```python
from build123d import *

# Parameters (mm, degrees)
SKETCH1_W           = 80
SKETCH1_H           = 80
BOSS_EXTRUDE1_DEPTH = 14
FILLET1_R           = 2
FILLET2_R           = 4
SKETCH2_R           = 5.75
CUT_EXTRUDE1_DEPTH  = 2
SKETCH3_R           = 1.5
CUT_EXTRUDE2_DEPTH  = 12
SKETCH6_R           = 6
CUT_EXTRUDE3_DEPTH  = 2
SKETCH7_W           = 33.5
SKETCH7_H           = 42
BOSS_EXTRUDE2_DEPTH = 2.5


with BuildPart() as part:
    # Sketch1 → Boss-Extrude1 (new, symmetric)
    with BuildSketch(Plane.XY):
        Rectangle(SKETCH1_W, SKETCH1_H)
    extrude(amount=BOSS_EXTRUDE1_DEPTH, both=True)

    # Fillet1
    fillet1_edges = [part.edges().sort_by_distance(p)[0] for p in [
        (-40, 0, 14),
        (0, -40, 14),
        (40, 0, 14),
        (0, 40, 14),
    ]]
    fillet(fillet1_edges, radius=FILLET1_R)

    # Fillet2
    # the kernel refuses this fillet: 4 mm, written as the material it takes off along each edge
    with BuildSketch(Plane(origin=(-36, -36, 14), x_dir=(-1, 0, 0), z_dir=(0, 1, 0))) as fillet2_piece_1:
        with BuildLine():
            CenterArc((2, -2), 2, 0, 90)
            Line((4, -2), (4, 0))
            Line((4, 0), (2, 0))
        make_face()
    revolve(axis=Axis((-36, -36, 14), (0, 0, 1)), revolution_arc=90, mode=Mode.SUBTRACT)
    with BuildSketch(Plane(origin=(-36, 36, 14), x_dir=(0, 1, 0), z_dir=(1, 0, 0))) as fillet2_piece_2:
        with BuildLine():
            CenterArc((2, -2), 2, 0, 90)
            Line((4, -2), (4, 0))
            Line((4, 0), (2, 0))
        make_face()
    revolve(axis=Axis((-36, 36, 14), (0, 0, 1)), revolution_arc=90, mode=Mode.SUBTRACT)
    with BuildSketch(Plane(origin=(36, -36, 14), x_dir=(0, -1, 0), z_dir=(-1, 0, 0))) as fillet2_piece_3:
        with BuildLine():
            CenterArc((2, -2), 2, 0, 90)
            Line((4, -2), (4, 0))
            Line((4, 0), (2, 0))
        make_face()
    revolve(axis=Axis((36, -36, 14), (0, 0, 1)), revolution_arc=90, mode=Mode.SUBTRACT)
    with BuildSketch(Plane(origin=(36, 36, 14), x_dir=(1, 0, 0), z_dir=(0, -1, 0))) as fillet2_piece_4:
        with BuildLine():
            CenterArc((2, -2), 2, 0, 90)
            Line((4, -2), (4, 0))
            Line((4, 0), (2, 0))
        make_face()
    revolve(axis=Axis((36, 36, 14), (0, 0, 1)), revolution_arc=90, mode=Mode.SUBTRACT)
    with BuildSketch(Plane(origin=(40, 40, 14), x_dir=(-1, 0, 0), z_dir=(0, 0, -1)), Plane(origin=(40, -40, 14), x_dir=(0, 1, 0), z_dir=(0, 0, -1)), Plane(origin=(-40, -40, -24), x_dir=(0, 1, 0), z_dir=(0, 0, 1)), Plane(origin=(-40, 40, -24), x_dir=(1, 0, 0), z_dir=(0, 0, 1))) as fillet2_piece_5:
        with BuildLine():
            CenterArc((FILLET2_R, -FILLET2_R), FILLET2_R, 90, 90)
            Line((0, -FILLET2_R), (0, 0))
            Line((0, 0), (FILLET2_R, 0))
        make_face()
    extrude(amount=38, mode=Mode.SUBTRACT)

    # Sketch2 → Cut-Extrude1 (cut)
    with BuildSketch(Plane.XY.offset(14)):
        with Locations((-27.6, 30.4)):
            Circle(SKETCH2_R)
        with Locations((-11.8, 30.4)):
            Circle(SKETCH2_R)
        with Locations((7.5, 30.4)):
            Circle(SKETCH2_R)
        with Locations((23.3, 30.4)):
            Circle(SKETCH2_R)
    extrude(amount=-CUT_EXTRUDE1_DEPTH, mode=Mode.SUBTRACT)

    # Sketch3 → Cut-Extrude2 (cut)
    with BuildSketch(Plane.XY.offset(14)):
        with Locations((-33.45, 21.95)):
            Circle(SKETCH3_R)
        with Locations((33.55, 21.95)):
            Circle(SKETCH3_R)
        with Locations((-33.45, -33.05)):
            Circle(SKETCH3_R)
        with Locations((33.55, -33.05)):
            Circle(SKETCH3_R)
    extrude(amount=-CUT_EXTRUDE2_DEPTH, mode=Mode.SUBTRACT)

    # Sketch6 → Cut-Extrude3 (cut)
    with BuildSketch(Plane.XY.offset(14)):
        with Locations((28.6, -16.4)):
            Circle(SKETCH6_R)
    extrude(amount=-CUT_EXTRUDE3_DEPTH, mode=Mode.SUBTRACT)

    # Sketch7 → Boss-Extrude2 (add)
    with BuildSketch(Plane(origin=(0, 0, -14), x_dir=(-1, 0, 0), z_dir=(0, 0, -1))):
        Rectangle(SKETCH7_W, SKETCH7_H)
    extrude(amount=BOSS_EXTRUDE2_DEPTH)


solid = part.part
```
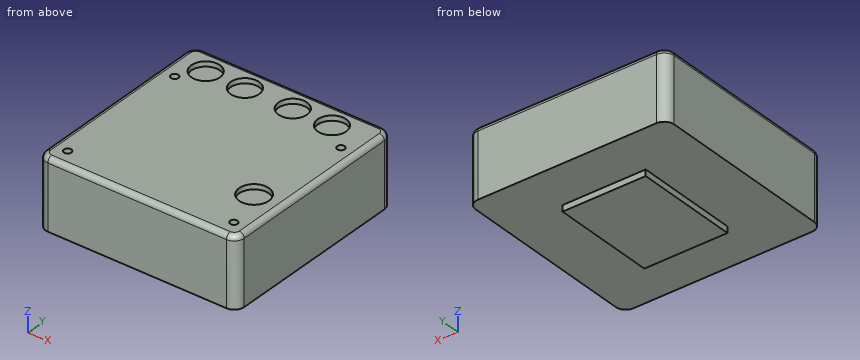
Geometry check sheet. Reference: the model listing, model coordinates, mm. Round coordinates to 2 decimals unless told otherwise and drop trailing zeros. Order: outer loops, then holes, each group sorted by start corner. A loop starts at its lowest first (then second) coordinate and runs counter-clockwise, first axis right, second up. Notation, with made-up numbers: (55.25, 46.25) - (68.25, 46.25) arc R19 cw to (68.25, 59.25) - close; hole circle Ø3 at (-15, -36). An arc over 180 degrees is marked (long way). Use a Markdown table: item, result. Add a question column.
1) Section check B-B (y = 5.5). Record the cut outline in (x, z).
2) Section check A-A (x = -4). Record the cut outline in (y, z), then the cut area to 3 significant figures.
3) Section check D-D (y = -16.4). Record the cut outline in (x, z), then the cut area to 3 significant figures.
4) Gauge pin test, flat ends, axial feed: P1, Ø4, axis at x = 33.55, y = -33.05, coming from the -Z side; P2, Ø7, axis at x = 23.3, y = 30.4, coming from the +Z side; P3, Ø1.5, axis at x = 33, y = -33.5, coming from the +Z side. Record the tip position at first contact, or that the pin passes through.
5) Thickness scan on line 1 along Y through (x, z) = (-33.45, 5.75); line 2 along X through (y, z) = (21, 5); line 3 along Z through (x, y) = (31.5, 17.5). Record the ranges inside material, lowest first.
6) Section check C-C (x = 7.5). Record the cut outline in (y, z), then the cut area to 3 significant figures.
Established:
| question | item | result |
|---|---|---|
| 1 | outline | (-40, -14) - (-16.75, -14) - (-16.75, -16.5) - (16.75, -16.5) - (16.75, -14) - (40, -14) - (40, 12) arc R2 ccw to (38, 14) - (-38, 14) arc R2 ccw to (-40, 12) - close |
| 2 | outline | (-40, -14) - (-21, -14) - (-21, -16.5) - (21, -16.5) - (21, -14) - (40, -14) - (40, 12) arc R2 ccw to (38, 14) - (-38, 14) arc R2 ccw to (-40, 12) - close |
| 2 | area | 2,340 mm2 |
| 3 | outline | (-40, -14) - (-16.75, -14) - (-16.75, -16.5) - (16.75, -16.5) - (16.75, -14) - (40, -14) - (40, 12) arc R2 ccw to (38, 14) - (34.6, 14) - (34.6, 12) - (22.6, 12) - (22.6, 14) - (-38, 14) arc R2 ccw to (-40, 12) - close |
| 3 | area | 2,300 mm2 |
| 4 | P1 | z = -14 |
| 4 | P2 | z = 12 |
| 4 | P3 | z = 2 |
| 5 | line 1 | -40 to -34.55, -31.55 to 20.45, 23.45 to 40 |
| 5 | line 2 | -40 to -34.61, -32.29 to 32.39, 34.71 to 40 |
| 5 | line 3 | -14 to 14 |
| 6 | outline | (-40, -14) - (-21, -14) - (-21, -16.5) - (21, -16.5) - (21, -14) - (40, -14) - (40, 12) arc R2 ccw to (38, 14) - (36.15, 14) - (36.15, 12) - (24.65, 12) - (24.65, 14) - (-38, 14) arc R2 ccw to (-40, 12) - close |
| 6 | area | 2,320 mm2 |
